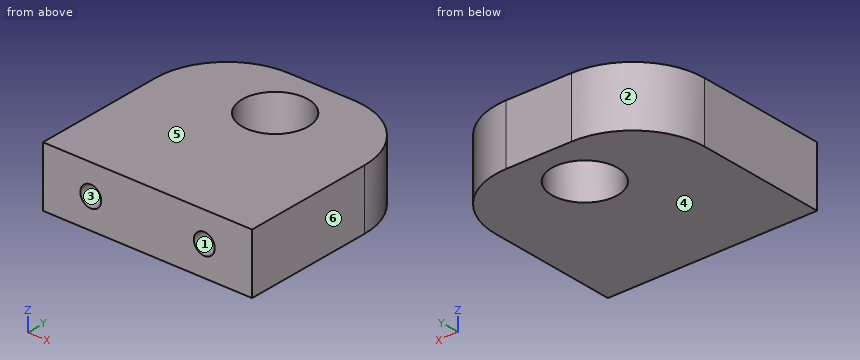
from build123d import *

# Parameters (mm, degrees)
SKETCH1_W           = 35
SKETCH1_H           = 10
BOSS_EXTRUDE1_DEPTH = 34
SKETCH2_R           = 5.5
CUT_EXTRUDE1_DEPTH  = 11
SKETCH3_R           = 1.75
CUT_EXTRUDE2_DEPTH  = 10
FILLET1_R           = 12


with BuildPart() as part:
    # Sketch1 → Boss-Extrude1 (new body)
    with BuildSketch(Plane(origin=(0, 0, 0), x_dir=(1, 0, 0), z_dir=(0, 1, 0))):
        with Locations((1.164675851, 4.144829176)):
            Rectangle(SKETCH1_W, SKETCH1_H)
    extrude(amount=BOSS_EXTRUDE1_DEPTH)

    # Sketch2 → Cut-Extrude1 (cut, through all)
    with BuildSketch(Plane.XY.offset(0.855170824)):
        with Locations((1.164675851, 25)):
            Circle(SKETCH2_R)
    extrude(amount=-CUT_EXTRUDE1_DEPTH, mode=Mode.SUBTRACT)

    # Sketch3 → Cut-Extrude2 (cut)
    with BuildSketch(Plane.XZ):
        with Locations((-8.335324149, -4.144829176)):
            Circle(SKETCH3_R)
        with Locations((10.664675851, -4.144829176)):
            Circle(SKETCH3_R)
    extrude(amount=-CUT_EXTRUDE2_DEPTH, mode=Mode.SUBTRACT)

    # Fillet1
    fillet1_edges = [part.edges().sort_by_distance(p)[0] for p in [
        (18.664675851, 34, -4.144829176),
        (-16.335324149, 34, -4.144829176),
    ]]
    fillet(fillet1_edges, radius=FILLET1_R)


solid = part.part
The model under review builds one solid part; all positions refer to its coordinate system, in mm. Face numbers are marked on the shaded views. A direction names the side the tool comes from. Coordinates: 2 decimals unless noted, no trailing zeros. Write each loop counter-clockwise with the first axis right and the second up, starting at its lowest first coordinate (ties: lowest second). Pieces come first, ordered by that corner, then holes. Notation, with made-up numbers: (-28, 18) - (-21, 18) arc R10 cw to (-21, 29) - close; hole circle Ø2 at (-27.5, 83). An arc over 180 degrees is marked (long way). Answer as a JSON object with one key per item and string values. Group by question number.
1. Add section A-A (x = 0). Give the boundary of the cut face in (y, z), plus the area to 3 significant figures.
2. Add section C-C (y = 8). Give the boundary of the cut face in (x, z), plus the area to 3 significant figures.
3. Mouldability with a two-part tool opening along Z and no side actions: class the marked faces 3, 4, 5 and 6 as pulls with the +Z half, pulls with the -Z half, needs draft (parallel to the pull), parting line crosses it, or undercut.
4. Clearance check with flat-ended pins moving along their axes: pin 1 Ø2 at (x, z) = (10.66, -4.14) entering from +Y; pin 2 Ø1 at (x, z) = (-8.5, -5) entering from -Y; pin 3 Ø1.5 at (x, z) = (-10, -2.5) entering from +Y. State where each tip first meets the part, or that it passes through.
5. Add section B-B (y = 25). Give the boundary of the cut face in (x, z).
6. To check wall thickness, follow probe 1 along Y at (x, z) = (1, -7.25); probe 2 along X at (y, z) = (28.5, -2); probe 3 along X at (y, z) = (29.5, -2.75). State the ranges of each line that lie inside material, in increasing order.
7. Add section D-D (x = 16). Give the boundary of the cut face in (y, z).
8. Machinability: for the marked faces 1 and 2, which of the approach directions +Z, -Z, +X, -X, +Y, -Y give a long, thin tool a straight path to every point of the face, cutting with its end or side? Answer none if there is none.
Findings:
{
 "1": {"outline": "(0, -9.14) - (19.62, -9.14) - (19.62, 0.86) - (0, 0.86) - close; (30.38, -9.14) - (34, -9.14) - (34, 0.86) - (30.38, 0.86) - close", "area": "232 mm²"},
 "2": {"outline": "(-16.34, -9.14) - (18.66, -9.14) - (18.66, 0.86) - (-16.34, 0.86) - close; hole circle Ø3.5 at (-8.34, -4.14); hole circle Ø3.5 at (10.66, -4.14)", "area": "331 mm²"},
 "3": {"face 3": "undercut", "face 4": "pulls with the -Z half", "face 5": "pulls with the +Z half", "face 6": "needs draft"},
 "4": {"pin 1": "y = 33.62", "pin 2": "y = 10", "pin 3": "y = 32.95"},
 "5": {"outline": "(-15.95, -9.14) - (-4.34, -9.14) - (-4.34, 0.86) - (-15.95, 0.86) - close; (6.66, -9.14) - (18.28, -9.14) - (18.28, 0.86) - (6.66, 0.86) - close"},
 "6": {"probe 1": "0 to 19.5, 30.5 to 34", "probe 2": "-14.42 to -3.08, 5.41 to 16.75", "probe 3": "-13.7 to -2, 4.33 to 16.03"},
 "7": {"outline": "(0, -9.14) - (29.54, -9.14) - (29.54, 0.86) - (0, 0.86) - close"},
 "8": {"face 1": "-Y", "face 2": "+Z, -Z, -X, +Y"}
}
